Read the model definition and answer for the solid it produces. Units are mm, in the model's axes. A direction names the side the tool comes from. Coordinates: 2 decimals unless noted, no trailing zeros. Loops run counter-clockwise (first coordinate to the right, second up) from the corner with the lowest first, then second, coordinate; pieces in that order, holes last. Notation, with made-up numbers: M 70.5,-28 L 125.5,-28 A22 ccw 125.5,-21 Z; hole C 48,57 d2. An arc over 180 degrees is marked long. One line per item, written item: value. Start each with the question number.
1. The part is cut by section D-D (x = -34). Write down the section's boundary in (y, z), then the cut area to 3 significant figures.
2. The part is cut by section C-C (y = -2.5). Write down the section's boundary in (x, z).
3. Determine the mould class of faces 1 (the face through (23.93, 0.75, 3.59)), 2 (the face through (-40.45, -6.38, 2.28)), 3 (the face through (41.72, -2, 2)) for opening direction Y: +Y half, -Y half, draft (parallel to the pull), parting line (faces both ways), or undercut.
4. A flat-ended cylindrical pin translates along its axis: pin 1 (2 mm diameter, centred on x = 32, y = -1, fed in from +Z). Find the tip coordinate at first contact, or state that the pin passes through.
5. The part is cut by section A-A (x = -25.5). Write down the section's boundary in (y, z), then the cut area to 3 significant figures.
6. The part is cut by section B-B (z = 3.45). Write down the section's boundary in (x, y).
7. Consider probe 1 along X at (y, z) = (1.75, 2.2); probe 2 along X at (y, z) = (-1, 3.35); probe 3 along X at (y, z) = (-2.75, 3.8). Determine where each line is inside the solid, lowest interval first.
8. For faces 4 (the face through (31.03, 0.23, 2.92)), 5 (the face through (-27, 3, 2.7)), 6 (the face through (-41.72, -2, 2)), determine the directions among +Z, -Z, +X, -X, +Y, -Y from which every point of the face is accessible in a straight line to the end or side of a thin tool.
```python
from build123d import *

# Parameters (mm, degrees)
SKETCH1_W            = 92
SKETCH1_H            = 75
BOSS_EXTRUDE1_DEPTH  = 4.5
M4_CLEARANCE_HOLE1_D = 4.5
M3_CLEARANCE_HOLE1_D = 3.4
CUT_EXTRUDE1_DEPTH   = 3.2
CUT_EXTRUDE2_DEPTH   = 2.7
SKETCH10_W           = 92
SKETCH10_H           = 29.25
SKETCH10_H_2         = 28.3
CUT_EXTRUDE3_DEPTH   = 60.51890456
CUT_EXTRUDE4_DEPTH   = 10


with BuildPart() as part:
    # Sketch1 → Boss-Extrude1 (new body)
    with BuildSketch(Plane.XY):
        Rectangle(SKETCH1_W, SKETCH1_H)
    extrude(amount=BOSS_EXTRUDE1_DEPTH)

    # M4 Clearance Hole1 (through all)
    with Locations(Plane.XY.offset(4.5)):
        with Locations((-34.669877487, -1.6), (34.130122513, -1.6)):
            Hole(M4_CLEARANCE_HOLE1_D / 2)

    # M3 Clearance Hole1 (through all)
    with Locations(Plane.XY.offset(4.5)):
        with Locations((-25.5, 1.4), (25.5, 1.4)):
            Hole(M3_CLEARANCE_HOLE1_D / 2)

    # Sketch8 → Cut-Extrude1 (cut)
    with BuildSketch(Plane.XY.offset(4.5)):
        Polygon((-30.512955548, -1.6), (-32.591416518, 2), (-36.748338456, 2), (-38.826799425, -1.6), (-36.748338456, -5.2), (-32.591416518, -5.2), align=None)
        Polygon((29.973200575, -1.6), (32.051661544, -5.2), (36.208583482, -5.2), (38.287044452, -1.6), (36.208583482, 2), (32.051661544, 2), align=None)
    extrude(amount=-CUT_EXTRUDE1_DEPTH, mode=Mode.SUBTRACT)

    # Sketch9 → Cut-Extrude2 (cut)
    with BuildSketch(Plane(origin=(0, 0, 0), x_dir=(-1, 0, 0), z_dir=(0, 0, -1))):
        Polygon((-22.209103466, 1.4), (-23.854551733, 4.25), (-27.145448267, 4.25), (-28.790896534, 1.4), (-27.145448267, -1.45), (-23.854551733, -1.45), align=None)
        Polygon((22.209103466, 1.4), (23.854551733, -1.45), (27.145448267, -1.45), (28.790896534, 1.4), (27.145448267, 4.25), (23.854551733, 4.25), align=None)
    extrude(amount=-CUT_EXTRUDE2_DEPTH, mode=Mode.SUBTRACT)

    # Sketch10 → Cut-Extrude3 (cut, through all)
    with BuildSketch(Plane(origin=(0, 0, 0), x_dir=(-1, 0, 0), z_dir=(0, 0, -1))):
        with Locations((0, 22.875)):
            Rectangle(SKETCH10_W, SKETCH10_H)
        with Locations((0, -23.35)):
            Rectangle(SKETCH10_W, SKETCH10_H_2)
    extrude(amount=-CUT_EXTRUDE3_DEPTH, mode=Mode.SUBTRACT)

    # Sketch11 → Cut-Extrude4 (cut)
    with BuildSketch(Plane.XY.offset(4.5)):
        Polygon((-39.13939839, 5.45), (-41.719877487, 0.980479097), (-41.719877487, -4.180479097), (-39.13939839, -8.65), (0, -8.65), (0, -18.65), (-51, -18.65), (-51, 15.45), (0, 15.45), (0, 5.45), align=None)
    cut_extrude4 = extrude(amount=-CUT_EXTRUDE4_DEPTH, mode=Mode.SUBTRACT)

    # Mirror1: Cut-Extrude4 across plane
    add(cut_extrude4.mirror(Plane(origin=(0, 0, 0), x_dir=(0, 0, 1), z_dir=(1, 0, 0))), mode=Mode.SUBTRACT)


solid = part.part
```
Answer block:
1. outline: M -8.65,0 L -3.75,0 L -3.75,1.3 L -5.2,1.3 L -5.2,4.5 L -8.65,4.5 Z; M 0.55,0 L 5.45,0 L 5.45,4.5 L 2,4.5 L 2,1.3 L 0.55,1.3 Z
1. area: 34.8 mm2
2. outline: M -41.72,0 L -36.73,0 L -36.73,1.3 L -38.31,1.3 L -38.31,4.5 L -41.72,4.5 Z; M -32.61,0 L 32.07,0 L 32.07,1.3 L 30.49,1.3 L 30.49,4.5 L -31.03,4.5 L -31.03,1.3 L -32.61,1.3 Z; M 36.19,0 L 41.72,0 L 41.72,4.5 L 37.77,4.5 L 37.77,1.3 L 36.19,1.3 Z
3. face 1: undercut
3. face 2: -Y half
3. face 3: draft
4. pin 1: stops at z = 1.3
5. outline: M -8.65,0 L -1.45,0 L -1.45,2.7 L -0.3,2.7 L -0.3,4.5 L -8.65,4.5 Z; M 3.1,2.7 L 4.25,2.7 L 4.25,0 L 5.45,0 L 5.45,4.5 L 3.1,4.5 Z
5. area: 41.9 mm2
6. outline: M -41.72,-4.18 L -39.14,-8.65 L 39.14,-8.65 L 41.72,-4.18 L 41.72,0.98 L 39.14,5.45 L -39.14,5.45 L -41.72,0.98 Z; hole M -38.83,-1.6 L -36.75,-5.2 L -32.59,-5.2 L -30.51,-1.6 L -32.59,2 L -36.75,2 Z; hole C -25.5,1.4 d3.4; hole C 25.5,1.4 d3.4; hole M 29.97,-1.6 L 32.05,-5.2 L 36.21,-5.2 L 38.29,-1.6 L 36.21,2 L 32.05,2 Z
7. probe 1: x = -41.28 to -36.89, -32.45 to -28.59, -22.41 to 22.41, 28.59 to 31.91, 36.35 to 41.28
7. probe 2: x = -41.72 to -38.48, -30.86 to 30.32, 37.94 to 41.72
7. probe 3: x = -41.72 to -38.16, -31.18 to 30.64, 37.62 to 41.72
8. face 4: +Z
8. face 5: -Z
8. face 6: +Z, -Z, -X, +Y, -Y
